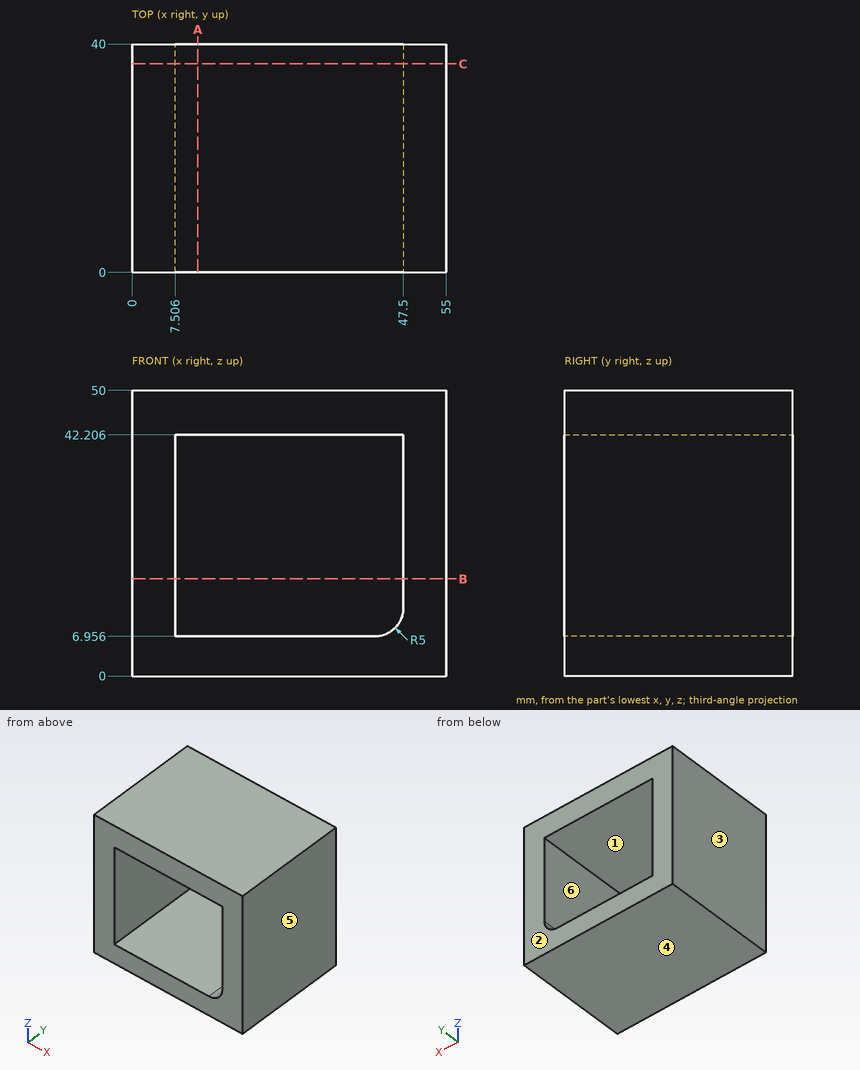
The drawing under review shows one solid part. Ordinate dimensions are in mm from its lowest x, y, z. A direction names the side the tool comes from. Round coordinates to 2 decimals unless told otherwise and drop trailing zeros. Loops run counter-clockwise (first coordinate to the right, second up) from the corner with the lowest first, then second, coordinate; pieces in that order, holes last. Notation, with made-up numbers: M 2,69.25 L 51,69.25 A9 cw 51,82.25 Z; hole C -25.75,-28.5 d9. An arc over 180 degrees is marked long. Answer as CSV lines item,"result". Start each with the question number.
Item 1: Consider section C-C (y = 36.5). Write out the cut boundary in (x, z).
Item 2: Insertion check: P1, Ø12, axis at x = 16, z = 20.5, coming from the +Y side; P2, Ø3, axis at y = 20, z = 15.5, coming from the -X side. Each pin has a flat end and moves straight along its axis. Give the tip position at first contact, or say it passes through.
Item 3: Consider section B-B (z = 17). Write out the cut boundary in (x, y), then the cut area to 3 significant figures.
Item 4: Mouldability with a two-part tool opening along X and no side actions: class the marked faces 3, 4, 5 and 6 as released by +X, released by -X, zero draft, split by the parting line, or undercut.
Item 5: For the marked faces 1 and 2, list the 3-axis set-ups (+Z, -Z, +X, -X, +Y, -Y) from which the entire face can be reached by the end or side of a thin tool; tool diameter is ignored.
Item 6: Consider section A-A (x = 11.5). Write out the cut boundary in (y, z).
Item 7: Wall thickness on line 1 (Z direction, x = 34.5, y = 15); line 2 (X direction, y = 2, z = 31.5); line 3 (X direction, y = 19.5, z = 9) (1 decimal): over which ranges is each line inside the solid? List them lowest first. Write a range as [from, to].
Answer:
1,outline,"M 0,0 L 55,0 L 55,50 L 0,50 Z; hole M 7.51,6.96 L 42.5,6.96 A5 ccw 47.5,11.96 L 47.5,42.21 L 7.51,42.21 Z"
2,P1,"passes through"
2,P2,"stops at x = 0"
3,outline,"M 0,0 L 7.51,0 L 7.51,40 L 0,40 Z; M 47.5,0 L 55,0 L 55,40 L 47.5,40 Z"
3,area,"600 mm^2"
4,face 3,"released by -X"
4,face 4,"zero draft"
4,face 5,"released by +X"
4,face 6,"undercut"
5,face 1,"+Y, -Y"
5,face 2,"+Z, -Z, +X, -X, +Y"
6,outline,"M 0,0 L 40,0 L 40,6.96 L 0,6.96 Z; M 0,42.21 L 40,42.21 L 40,50 L 0,50 Z"
7,line 1,"z = [0, 6.96], [42.21, 50]"
7,line 2,"x = [0, 7.51], [47.5, 55]"
7,line 3,"x = [0, 7.5], [46.5, 55]"
